Read the model definition and answer for the solid it produces. Units are mm, in the model's axes. A direction names the side the tool comes from. Coordinates: 2 decimals unless noted, no trailing zeros. Order: outer loops, then holes, each group sorted by start corner. A loop starts at its lowest first (then second) coordinate and runs counter-clockwise, first axis right, second up. Notation, with made-up numbers: M -13.5,-6 L 25.5,-6 A25 ccw 25.5,10 Z; hole C 27,71.5 d7. An arc over 180 degrees is marked long. Put each result on its own line as item: value.
from build123d import *

# Parameters (mm, degrees)
F0_R     = 3
F1_DEPTH = 10


with BuildPart() as f1:
    # F0 (on Front) → F1 (new body)
    with BuildSketch(Plane.XZ):
        with BuildLine():
            ThreePointArc((8.523458, -1.144846), (8.580843, -0.573701), (8.6, 0))
            ThreePointArc((8.6, 0), (8.594903, 0.296051), (8.579617, 0.59175))
            ThreePointArc((8.579617, 0.59175), (8.26071, 2.391793), (7.568545, 4.083763))
            ThreePointArc((7.568545, 4.083763), (7.117297, 4.82743), (6.593234, 5.521708))
            ThreePointArc((6.593234, 5.521708), (5.277194, 6.790524), (3.722706, 7.752513))
            ThreePointArc((3.722706, 7.752513), (2.920522, 8.088915), (2.08846, 8.342562))
            ThreePointArc((2.08846, 8.342562), (0.27797, 8.595507), (-1.54508, 8.460067))
            ThreePointArc((-1.54508, 8.460067), (-2.391793, 8.26071), (-3.214035, 7.97684))
            ThreePointArc((-3.214035, 7.97684), (-4.82743, 7.117297), (-6.222699, 5.936162))
            ThreePointArc((-6.222699, 5.936162), (-6.790524, 5.277194), (-7.288878, 4.564237))
            ThreePointArc((-7.288878, 4.564237), (-8.088915, 2.920522), (-8.523458, 1.144846))
            ThreePointArc((-8.523458, 1.144846), (-8.595507, 0.27797), (-8.579617, -0.59175))
            ThreePointArc((-8.579617, -0.59175), (-8.26071, -2.391793), (-7.568545, -4.083763))
            ThreePointArc((-7.568545, -4.083763), (-7.117297, -4.82743), (-6.593234, -5.521708))
            ThreePointArc((-6.593234, -5.521708), (-5.277194, -6.790524), (-3.722706, -7.752513))
            ThreePointArc((-3.722706, -7.752513), (-2.920522, -8.088915), (-2.08846, -8.342562))
            ThreePointArc((-2.08846, -8.342562), (-0.27797, -8.595507), (1.54508, -8.460067))
            ThreePointArc((1.54508, -8.460067), (2.391793, -8.26071), (3.214035, -7.97684))
            ThreePointArc((3.214035, -7.97684), (4.82743, -7.117297), (6.222699, -5.936162))
            ThreePointArc((6.222699, -5.936162), (6.790524, -5.277194), (7.288878, -4.564237))
            ThreePointArc((7.288878, -4.564237), (8.088915, -2.920522), (8.523458, -1.144846))
        make_face()
        Circle(F0_R, mode=Mode.SUBTRACT)
        with BuildLine():
            ThreePointArc((7.568545, 4.083763), (8.26071, 2.391793), (8.579617, 0.59175))
            ThreePointArc((8.579617, 0.59175), (8.678841, 0.926698), (8.973122, 1.114938))
            Line((8.973122, 1.114938), (11.383292, 1.634219))
            ThreePointArc((11.383292, 1.634219), (9.509422, 2.753343), (10.495478, 4.700525))
            Line((10.495478, 4.700525), (8.180708, 3.851754))
            ThreePointArc((8.180708, 3.851754), (7.831378, 3.853644), (7.568545, 4.083763))
        make_face()
        with BuildLine():
            ThreePointArc((8.882336, -1.692365), (8.600833, -1.485505), (8.523458, -1.144846))
            ThreePointArc((8.523458, -1.144846), (8.088915, -2.920522), (7.288878, -4.564237))
            ThreePointArc((7.288878, -4.564237), (7.566029, -4.35158), (7.914752, -4.372265))
            Line((7.914752, -4.372265), (10.169846, -5.36882))
            ThreePointArc((10.169846, -5.36882), (9.311658, -3.361997), (11.25392, -2.366283))
            Line((11.25392, -2.366283), (8.882336, -1.692365))
        make_face()
        with BuildLine():
            ThreePointArc((3.722706, 7.752513), (5.277194, 6.790524), (6.593234, 5.521708))
            ThreePointArc((6.593234, 5.521708), (6.47663, 5.851009), (6.604064, 6.176272))
            Line((6.604064, 6.176272), (8.248707, 8.013042))
            ThreePointArc((8.248707, 8.013042), (6.07491, 7.816999), (5.728121, 9.971892))
            Line((5.728121, 9.971892), (4.354328, 7.924634))
            ThreePointArc((4.354328, 7.924634), (4.070602, 7.720832), (3.722706, 7.752513))
        make_face()
        with BuildLine():
            ThreePointArc((10.495478, 4.700525), (9.509422, 2.753343), (11.383292, 1.634219))
            ThreePointArc((11.383292, 1.634219), (12.291125, 2.193138), (12.646298, 3.198328))
            ThreePointArc((12.646298, 3.198328), (11.962455, 4.510065), (10.495478, 4.700525))
        make_face()
        with BuildLine():
            ThreePointArc((6.191214, -6.590058), (6.085062, -6.257241), (6.222699, -5.936162))
            ThreePointArc((6.222699, -5.936162), (4.82743, -7.117297), (3.214035, -7.97684))
            ThreePointArc((3.214035, -7.97684), (3.563252, -7.967703), (3.833216, -8.189411))
            Line((3.833216, -8.189411), (5.071865, -10.321152))
            ThreePointArc((5.071865, -10.321152), (5.557158, -8.193168), (7.713746, -8.529251))
            Line((7.713746, -8.529251), (6.191214, -6.590058))
        make_face()
        with BuildLine():
            ThreePointArc((12.416573, -3.90535), (12.093239, -2.940921), (11.25392, -2.366283))
            ThreePointArc((11.25392, -2.366283), (9.311658, -3.361997), (10.169846, -5.36882))
            ThreePointArc((10.169846, -5.36882), (11.689853, -5.246014), (12.416573, -3.90535))
        make_face()
        with BuildLine():
            ThreePointArc((-1.54508, 8.460067), (0.27797, 8.595507), (2.08846, 8.342562))
            ThreePointArc((2.08846, 8.342562), (1.800567, 8.540434), (1.712478, 8.878481))
            Line((1.712478, 8.878481), (1.963396, 11.331155))
            ThreePointArc((1.963396, 11.331155), (0.319988, 9.894827), (-1.227184, 11.434335))
            Line((-1.227184, 11.434335), (-1.135258, 8.970573))
            ThreePointArc((-1.135258, 8.970573), (-1.245005, 8.638924), (-1.54508, 8.460067))
        make_face()
        with BuildLine():
            ThreePointArc((5.728121, 9.971892), (6.07491, 7.816999), (8.248707, 8.013042))
            ThreePointArc((8.248707, 8.013042), (8.551235, 8.509034), (8.656713, 9.080352))
            ThreePointArc((8.656713, 9.080352), (7.522681, 10.610997), (5.728121, 9.971892))
        make_face()
        with BuildLine():
            ThreePointArc((1.135258, -8.970573), (1.245005, -8.638924), (1.54508, -8.460067))
            ThreePointArc((1.54508, -8.460067), (-0.27797, -8.595507), (-2.08846, -8.342562))
            ThreePointArc((-2.08846, -8.342562), (-1.800567, -8.540434), (-1.712478, -8.878481))
            Line((-1.712478, -8.878481), (-1.963396, -11.331155))
            ThreePointArc((-1.963396, -11.331155), (-0.319988, -9.894827), (1.227184, -11.434335))
            Line((1.227184, -11.434335), (1.135258, -8.970573))
        make_face()
        with BuildLine():
            ThreePointArc((8.055284, -9.517316), (7.967491, -8.994602), (7.713746, -8.529251))
            ThreePointArc((7.713746, -8.529251), (5.557158, -8.193168), (5.071865, -10.321152))
            ThreePointArc((5.071865, -10.321152), (6.871535, -11.062222), (8.055284, -9.517316))
        make_face()
        with BuildLine():
            ThreePointArc((-6.222699, 5.936162), (-4.82743, 7.117297), (-3.214035, 7.97684))
            ThreePointArc((-3.214035, 7.97684), (-3.563252, 7.967703), (-3.833216, 8.189411))
            Line((-3.833216, 8.189411), (-5.071865, 10.321152))
            ThreePointArc((-5.071865, 10.321152), (-4.910378, 9.933567), (-4.855284, 9.517316))
            ThreePointArc((-4.855284, 9.517316), (-5.93257, 8.005109), (-7.713746, 8.529251))
            Line((-7.713746, 8.529251), (-6.191214, 6.590058))
            ThreePointArc((-6.191214, 6.590058), (-6.085062, 6.257241), (-6.222699, 5.936162))
        make_face()
        with BuildLine():
            ThreePointArc((-1.227184, 11.434335), (0.319988, 9.894827), (1.963396, 11.331155))
            ThreePointArc((1.963396, 11.331155), (1.969625, 11.412467), (1.971704, 11.493991))
            ThreePointArc((1.971704, 11.493991), (0.34187, 13.093713), (-1.227184, 11.434335))
        make_face()
        with BuildLine():
            ThreePointArc((-4.354328, -7.924634), (-4.070602, -7.720832), (-3.722706, -7.752513))
            ThreePointArc((-3.722706, -7.752513), (-5.277194, -6.790524), (-6.593234, -5.521708))
            ThreePointArc((-6.593234, -5.521708), (-6.47663, -5.851009), (-6.604064, -6.176272))
            Line((-6.604064, -6.176272), (-8.248707, -8.013042))
            ThreePointArc((-8.248707, -8.013042), (-6.485394, -7.585831), (-5.456713, -9.080352))
            ThreePointArc((-5.456713, -9.080352), (-5.526068, -9.546321), (-5.728121, -9.971892))
            Line((-5.728121, -9.971892), (-4.354328, -7.924634))
        make_face()
        with BuildLine():
            ThreePointArc((1.228296, -11.493991), (1.228018, -11.464158), (1.227184, -11.434335))
            ThreePointArc((1.227184, -11.434335), (-0.319988, -9.894827), (-1.963396, -11.331155))
            ThreePointArc((-1.963396, -11.331155), (-0.453228, -13.091913), (1.228296, -11.493991))
        make_face()
        with BuildLine():
            ThreePointArc((-8.523458, 1.144846), (-8.088915, 2.920522), (-7.288878, 4.564237))
            ThreePointArc((-7.288878, 4.564237), (-7.566029, 4.35158), (-7.914752, 4.372265))
            Line((-7.914752, 4.372265), (-10.169846, 5.36882))
            ThreePointArc((-10.169846, 5.36882), (-9.475908, 4.77863), (-9.216573, 3.90535))
            ThreePointArc((-9.216573, 3.90535), (-9.852144, 2.628683), (-11.25392, 2.366283))
            Line((-11.25392, 2.366283), (-8.882336, 1.692365))
            ThreePointArc((-8.882336, 1.692365), (-8.600833, 1.485505), (-8.523458, 1.144846))
        make_face()
        with BuildLine():
            ThreePointArc((-4.855284, 9.517316), (-4.910378, 9.933567), (-5.071865, 10.321152))
            ThreePointArc((-5.071865, 10.321152), (-7.353411, 10.841465), (-7.713746, 8.529251))
            ThreePointArc((-7.713746, 8.529251), (-5.93257, 8.005109), (-4.855284, 9.517316))
        make_face()
        with BuildLine():
            ThreePointArc((-8.180708, -3.851754), (-7.831378, -3.853644), (-7.568545, -4.083763))
            ThreePointArc((-7.568545, -4.083763), (-8.26071, -2.391793), (-8.579617, -0.59175))
            ThreePointArc((-8.579617, -0.59175), (-8.678841, -0.926698), (-8.973122, -1.114938))
            Line((-8.973122, -1.114938), (-11.383292, -1.634219))
            ThreePointArc((-11.383292, -1.634219), (-10.041109, -1.9535), (-9.446298, -3.198328))
            ThreePointArc((-9.446298, -3.198328), (-9.73456, -4.114485), (-10.495478, -4.700525))
            Line((-10.495478, -4.700525), (-8.180708, -3.851754))
        make_face()
        with BuildLine():
            ThreePointArc((-8.248707, -8.013042), (-8.038517, -10.343706), (-5.728121, -9.971892))
            ThreePointArc((-5.728121, -9.971892), (-5.526068, -9.546321), (-5.456713, -9.080352))
            ThreePointArc((-5.456713, -9.080352), (-6.485394, -7.585831), (-8.248707, -8.013042))
        make_face()
        with BuildLine():
            ThreePointArc((-9.216573, 3.90535), (-9.475908, 4.77863), (-10.169846, 5.36882))
            ThreePointArc((-10.169846, 5.36882), (-12.321487, 4.448703), (-11.25392, 2.366283))
            ThreePointArc((-11.25392, 2.366283), (-9.852144, 2.628683), (-9.216573, 3.90535))
        make_face()
        with BuildLine():
            ThreePointArc((-11.383292, -1.634219), (-12.583174, -3.643312), (-10.495478, -4.700525))
            ThreePointArc((-10.495478, -4.700525), (-9.73456, -4.114485), (-9.446298, -3.198328))
            ThreePointArc((-9.446298, -3.198328), (-10.041109, -1.9535), (-11.383292, -1.634219))
        make_face()
    extrude(amount=F1_DEPTH)


solid = f1.part
Q1. Find section A-A on x = 0. Write down the section's boundary in (y, z), plus the area to 3 significant figures.
Answers below:
outline: M -10,-13.05 L 0,-13.05 L 0,-3 L -10,-3 Z; M -10,3 L 0,3 L 0,13.05 L -10,13.05 Z
area: 201 mm^2
Q2. A tool of negligible diameter and unlimited length cuts with its end or side. For faces 4 (the face through (-2.932, -4.93, -8.085)), 5 (the face through (-1.18, -4.93, 10.22)), 6 (the face through (5.05, -4.93, 8.96)), 7 (the face through (3, 0, 3)), 8 (the face through (-7.415, -4.93, -7.082)), from which of +Z, -Z, +X, -X, +Y, -Y can it reach the whole face along a straight path? Write none if from no direction.
Answers below:
face 4: -Z, +Y, -Y
face 5: +Y, -Y
face 6: +Z, +Y, -Y
face 7: +Z, -Z, +X, -X, +Y
face 8: -X, +Y, -Y
Q3. Given pin 1 (2 mm diameter, centred on x = -3, y = -3, fed in from +Z); pin 2 (2 mm diameter, centred on x = 3, y = -3, fed in from -Z), each flat-ended and moving along its own axis, determine where each tip first touches the part or whether it passes through.
Answers below:
pin 1: stops at z = 8.48
pin 2: stops at z = -8.48
Q4. For a pull along Z with two mould halves and no side action, classify faces 1 (the face through (-4.444, -4.93, 9.24)), 2 (the face through (2.38, -4.93, -8.264)), 3 (the face through (10.085, -4.93, -2.034)) as +Z half, -Z half, draft (parallel to the pull), parting line (faces both ways), or undercut.
Answers below:
face 1: +Z half
face 2: -Z half
face 3: undercut
Q5. Consider line 1 along X through (y, z) = (-2, -9.75); line 2 along X through (y, z) = (-6.75, 10.5); line 3 along Z through (x, y) = (-11, -5.25). Determine where each line is inside the solid, lowest interval first.
Answers below:
line 1: x = -8.51 to -5.58, -1.8 to 1.16, 4.74 to 8.04
line 2: x = -7.72 to -5.19, -1.19 to 1.88, 6.32 to 7.79
line 3: z = -4.8 to -1.55, 2.29 to 5.49
